The model under review builds one solid part; all positions refer to its coordinate system, in mm. A direction names the side the tool comes from. Round coordinates to 2 decimals unless told otherwise and drop trailing zeros. Order: outer loops, then holes, each group sorted by start corner. A loop starts at its lowest first (then second) coordinate and runs counter-clockwise, first axis right, second up. Notation, with made-up numbers: M 17.5,28 L 42.5,28 A22 cw 42.5,39 Z; hole C -13,-7 d5. An arc over 180 degrees is marked long. One line per item, written item: value. Start each with the question number.
from build123d import *

# Parameters (mm, degrees)
SKETCH1_R           = 2.4003
BOSS_EXTRUDE1_DEPTH = 0.1778
CIRPATTERN1_COUNT   = 3
SKETCH2_R           = 1.0033
CUT_EXTRUDE3_DEPTH  = 11.598193754
CIRPATTERN2_COUNT   = 3
FILLET1_R           = 2.54
BOSS_EXTRUDE2_START = -0.762
BOSS_EXTRUDE2_DEPTH = 0.762
CIRPATTERN3_COUNT   = 3


with BuildPart() as part:
    # Sketch1 → Boss-Extrude1 (new body)
    with BuildSketch(Plane(origin=(0, 0, 0), x_dir=(1, 0, 0), z_dir=(0, 1, 0))):
        with BuildLine():
            ThreePointArc((-2.080029721, 5.48099038), (-1.52284746, 5.377722752), (-1.27, 4.870589203))
            Line((-1.27, 4.870589203), (-1.27, 2.036796526))
            ThreePointArc((-1.27, 2.036796526), (0, 2.4003), (1.27, 2.036796526))
            Line((1.27, 2.036796526), (1.27, 4.870589203))
            ThreePointArc((1.27, 4.870589203), (1.52284746, 5.377722752), (2.080029721, 5.48099038))
            Line((2.080029721, 5.48099038), (5.363123917, 4.539578268))
            ThreePointArc((5.363123917, 4.539578268), (5.647788598, 4.647944118), (5.62377215, 4.951589221))
            ThreePointArc((5.62377215, 4.951589221), (0, 7.493), (-5.62377215, 4.951589221))
            ThreePointArc((-5.62377215, 4.951589221), (-5.647788598, 4.647944118), (-5.363123917, 4.539578268))
            Line((-5.363123917, 4.539578268), (-2.080029721, 5.48099038))
        make_face()
        Circle(SKETCH1_R)
    boss_extrude1 = extrude(amount=BOSS_EXTRUDE1_DEPTH)

    # CirPattern1: Boss-Extrude1 ×3 about axis
    cirpattern1_axis = Axis((0, 0, 0), (0, 1, 0))
    for i in range(1, CIRPATTERN1_COUNT):
        add(boss_extrude1.rotate(cirpattern1_axis, i * 360 / CIRPATTERN1_COUNT))

    # Sketch2 → Cut-Extrude3 (cut, through all)
    with BuildSketch(Plane(origin=(0, 0.1778, 0), x_dir=(1, 0, 0), z_dir=(0, 1, 0))):
        Circle(SKETCH2_R)
        with BuildLine():
            Line((0.3175, 0.951737695), (0.3175, 1.5367))
            Line((0.3175, 1.5367), (-0.3175, 1.5367))
            Line((-0.3175, 1.5367), (-0.3175, 0.951737695))
            ThreePointArc((-0.3175, 0.951737695), (0, 1.0033), (0.3175, 0.951737695))
        make_face()
    cut_extrude3 = extrude(amount=-CUT_EXTRUDE3_DEPTH, mode=Mode.SUBTRACT)

    # CirPattern2: Cut-Extrude3 ×3 about axis
    cirpattern2_axis = Axis((0, 0, 0), (0, 1, 0))
    for i in range(1, CIRPATTERN2_COUNT):
        add(cut_extrude3.rotate(cirpattern2_axis, i * 360 / CIRPATTERN2_COUNT), mode=Mode.SUBTRACT)

    # Fillet1
    fillet1_edges = [part.edges().sort_by_distance(p)[0] for p in [
        (1.27, 0.0889, -2.036796526),
        (-1.27, 0.0889, -2.036796526),
        (2.398917534, 0.0889, -0.081454),
        (-1.128917534, 0.0889, 2.118250526),
        (-2.398917534, 0.0889, -0.081454),
        (1.128917534, 0.0889, 2.118250526),
    ]]
    fillet(fillet1_edges, radius=FILLET1_R)

    # Sketch3 → Boss-Extrude2 (add)
    with BuildSketch(Plane(origin=(0, 0.1778, 0), x_dir=(1, 0, 0), z_dir=(0, 1, 0)).offset(BOSS_EXTRUDE2_START)):
        with BuildLine():
            Line((-4.980841253, 4.437807212), (-2.02402021, 5.285662003))
            ThreePointArc((-2.02402021, 5.285662003), (-1.645136273, 5.215440016), (-1.4732, 4.870589203))
            Line((-1.4732, 4.870589203), (-1.4732, 3.144910824))
            ThreePointArc((-1.4732, 3.144910824), (-1.610918341, 2.354547555), (-2.007840617, 1.65734375))
            ThreePointArc((-2.007840617, 1.65734375), (-2.254697139, 1.30175), (-2.439222099, 0.910169106))
            ThreePointArc((-2.439222099, 0.910169106), (-2.844557167, 0.217822429), (-3.460172666, -0.296626787))
            Line((-3.460172666, -0.296626787), (-4.954653981, -1.159465976))
            ThreePointArc((-4.954653981, -1.159465976), (-5.339271682, -1.182990203), (-5.589527676, -0.889978082))
            Line((-5.589527676, -0.889978082), (-6.33367441, 2.094631451))
            ThreePointArc((-6.33367441, 2.094631451), (-6.478847097, 2.366941647), (-6.73524563, 2.538661605))
            Line((-6.73524563, 2.538661605), (-6.773580549, 2.552424483))
            ThreePointArc((-6.773580549, 2.552424483), (-6.671021136, 2.4837365), (-6.612952061, 2.374812422))
            Line((-6.612952061, 2.374812422), (-5.786691767, -0.939136611))
            ThreePointArc((-5.786691767, -0.939136611), (-5.418668247, -1.370036789), (-4.853053981, -1.335442339))
            Line((-4.853053981, -1.335442339), (-3.358572666, -0.472603149))
            ThreePointArc((-3.358572666, -0.472603149), (-2.689425385, 0.086580782), (-2.248843789, 0.839131517))
            ThreePointArc((-2.248843789, 0.839131517), (-2.078720777, 1.20015), (-1.851131105, 1.527990092))
            ThreePointArc((-1.851131105, 1.527990092), (-1.419693849, 2.285820314), (-1.27, 3.144910824))
            Line((-1.27, 3.144910824), (-1.27, 4.870589203))
            ThreePointArc((-1.27, 4.870589203), (-1.52284746, 5.377722752), (-2.080029721, 5.48099038))
            Line((-2.080029721, 5.48099038), (-5.363123917, 4.539578268))
            ThreePointArc((-5.363123917, 4.539578268), (-5.486489473, 4.535405523), (-5.597254718, 4.589880588))
            Line((-5.597254718, 4.589880588), (-5.566168256, 4.563563014))
            ThreePointArc((-5.566168256, 4.563563014), (-5.289255144, 4.42737535), (-4.980841253, 4.437807212))
        make_face()
    boss_extrude2 = extrude(amount=BOSS_EXTRUDE2_DEPTH)

    # CirPattern3: Boss-Extrude2 ×3 about axis
    cirpattern3_axis = Axis((0, 0, 0), (0, 1, 0))
    for i in range(1, CIRPATTERN3_COUNT):
        add(boss_extrude2.rotate(cirpattern3_axis, i * 360 / CIRPATTERN3_COUNT))


solid = part.part
Item 1: Consider section A-A, the plane z = -1.25. Give the boundary of the cut face in (x, y), then the cut area to 3 significant figures.
Item 2: Consider section D-D, the plane z = -2.75. Give the boundary of the cut face in (x, y), then the cut area to 3 significant figures.
Item 3: Wall thickness on L1, parallel to X at y = -0.45, z = 0.75; L2, parallel to Z at x = 3.75, y = -0.2; L3, parallel to X at y = -0.4, z = -2: over which ranges is each line inside the solid? List them lowest first.
Item 4: Clearance check with a flat-ended pin moving along its axis: P1, Ø1.5, axis at x = 1.5, z = -0.5, coming from the -Y side. State where the tip first meets the part, or that it passes through.
Item 5: Consider section B-B, the plane y = -0.2. Count the separate pieces of the cut face and the enclosed holes in it, then the cut area to 3 significant figures.
Item 6: The part is to be moulded in two halves that separate along Z. For faces 5 (the flat face through (-2.44, -0.21, 5.48)), 6 (the flat face through (-2.495, -0.296, 5.712)), 7 (the flat face through (3.745, -0.296, -5.004)), say which applies: pulls with the +Z half, pulls with the -Z half, needs draft (parallel to the pull), parting line crosses it, or undercut.
Item 7: Consider section C-C, the plane z = 4.75. Give the boundary of the cut face in (x, y), then the cut area to 3 significant figures.
Item 8: Machinability: for faces 1 (the flat face through (4.218, -0.209, 0.734)), 2 (the flat face through (-6.206, -0.296, -0.741)), 3 (the flat face through (4.1, -0.3, 0.9)), 4 (the flat face through (-2.83, -0.3, 3.1)), which of the approach directions +Z, -Z, +X, -X, +Y, -Y give a long, thin tool a straight path to every point of the face, cutting with its end or side? Answer none if there is none.
Computed:
1. outline: M -7.39,0 L -6.33,0 L -6.33,-0.58 L -6.12,-0.58 L -6.12,0.18 L -7.39,0.18 Z; M -2.28,-0.58 L -2.05,-0.58 L -2.05,0 L -0.32,0 L -0.32,0.18 L -2.28,0.18 Z; M 0.32,0 L 2.05,0 L 2.05,-0.58 L 2.28,-0.58 L 2.28,0.18 L 0.32,0.18 Z; M 6.12,-0.58 L 6.33,-0.58 L 6.33,0 L 7.39,0 L 7.39,0.18 L 6.12,0.18 Z
1. area: 1.67 mm^2
2. outline: M -1.51,-0.58 L -1.3,-0.58 L -1.3,0 L 1.3,0 L 1.3,-0.58 L 1.51,-0.58 L 1.51,0.18 L -1.51,0.18 Z
2. area: 0.776 mm^2
3. L1: x = -5.83 to -5.62, -4.25 to -3.84, 3.84 to 4.25, 5.62 to 5.83
3. L2: z = -5 to -4.79, 0.46 to 0.7, 3.67 to 4.5
3. L3: x = -6.52 to -6.31, -1.77 to -1.54, 1.54 to 1.77, 6.31 to 6.52
4. P1: stops at y = 0
5. separate pieces: 3
5. enclosed holes: 0
5. area: 10.0 mm^2
6. face 5: undercut
6. face 6: pulls with the +Z half
6. face 7: pulls with the -Z half
7. outline: M -5.8,0 L -3.49,0 L -3.49,-0.58 L -3.2,-0.58 L -3.2,0.18 L -5.8,0.18 Z; M 3.2,-0.58 L 3.49,-0.58 L 3.49,0 L 5.8,0 L 5.8,0.18 L 3.2,0.18 Z
7. area: 1.27 mm^2
8. face 1: +Y, -Y
8. face 2: +Z, -X, -Y
8. face 3: -Y
8. face 4: -X, -Y
